Input: dimensioned drawing with shaded views. Units: mm. Origin: part minimum x, y, z. A direction names the side the tool comes from. Round coordinates to 2 decimals unless told otherwise and drop trailing zeros. Order: outer loops, then holes, each group sorted by start corner. A loop starts at its lowest first (then second) coordinate and runs counter-clockwise, first axis right, second up.
Item 1: Cut plane D-D on z = 70. Output: boundary loops of the cut face in (x, y).
Item 2: Reachability of the marked faces 1 and 2 from +Z, -Z, +X, -X, +Y, -Y: full face, straight path, thin tool, end or side. Return the list, or none.
Item 3: Line query: L1, parallel to Y at x = 1, z = 70; L2, parallel to Z at x = 1.9, y = 20; L3, parallel to X at y = 30, z = 1. Output: solid intervals per line, ascending.
Item 4: Cut plane A-A on z = 50. Output: boundary loops of the cut face in (x, y), then the cut area to 3 significant figures.
Item 5: First-contact query: pin 1 (3.5 mm diameter, centred on x = 30, y = 50, fed in from +Z); pin 2 (3 mm diameter, centred on x = 66.5, y = 19, fed in from -Z); pin 3 (6.5 mm diameter, centred on x = 30, y = 30, fed in from +Z); pin 4 (5 mm diameter, centred on y = 70, z = 70, fed in from +X). Flat tips, straight axial feed; report the tip coordinate or a pass-through.
Item 6: Cut plane C-C on x = 30. Output: boundary loops of the cut face in (y, z).
Item 7: Cut plane B-B on y = 30. Output: boundary loops of the cut face in (x, z), then the cut area to 3 significant figures.
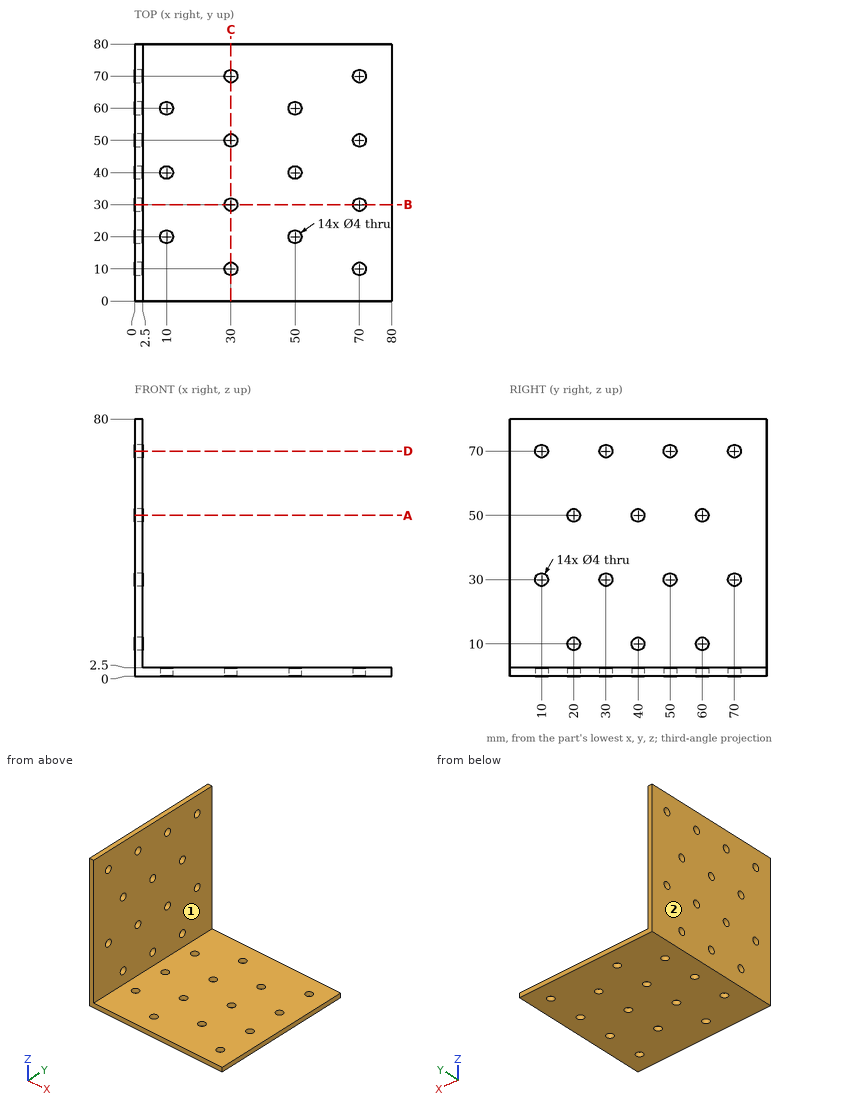
From the geometry:
1. outline: (0, 0) - (2.5, 0) - (2.5, 8) - (0, 8) - close; (0, 12) - (2.5, 12) - (2.5, 28) - (0, 28) - close; (0, 32) - (2.5, 32) - (2.5, 48) - (0, 48) - close; (0, 52) - (2.5, 52) - (2.5, 68) - (0, 68) - close; (0, 72) - (2.5, 72) - (2.5, 80) - (0, 80) - close
2. face 1: +Z, +X, +Y, -Y
2. face 2: +Z, -Z, -X, +Y, -Y
3. L1: y = 0 to 8, 12 to 28, 32 to 48, 52 to 68, 72 to 80
3. L2: z = 0 to 8, 12 to 48, 52 to 80
3. L3: x = 0 to 28, 32 to 68, 72 to 80
4. outline: (0, 0) - (2.5, 0) - (2.5, 18) - (0, 18) - close; (0, 22) - (2.5, 22) - (2.5, 38) - (0, 38) - close; (0, 42) - (2.5, 42) - (2.5, 58) - (0, 58) - close; (0, 62) - (2.5, 62) - (2.5, 80) - (0, 80) - close
4. area: 170 mm2
5. pin 1: passes through
5. pin 2: stops at z = 0
5. pin 3: stops at z = 2.5
5. pin 4: stops at x = 2.5
6. outline: (0, 0) - (8, 0) - (8, 2.5) - (0, 2.5) - close; (12, 0) - (28, 0) - (28, 2.5) - (12, 2.5) - close; (32, 0) - (48, 0) - (48, 2.5) - (32, 2.5) - close; (52, 0) - (68, 0) - (68, 2.5) - (52, 2.5) - close; (72, 0) - (80, 0) - (80, 2.5) - (72, 2.5) - close
7. outline: (0, 0) - (28, 0) - (28, 2.5) - (2.5, 2.5) - (2.5, 28) - (0, 28) - close; (0, 32) - (2.5, 32) - (2.5, 68) - (0, 68) - close; (0, 72) - (2.5, 72) - (2.5, 80) - (0, 80) - close; (32, 0) - (68, 0) - (68, 2.5) - (32, 2.5) - close; (72, 0) - (80, 0) - (80, 2.5) - (72, 2.5) - close
7. area: 354 mm2
